Autodesk Inventor part; units mm, degrees
ref_plane "YZ Plane" through (0, 0, 0) normal (1, 0, 0) x (0, 1, 0)
ref_plane "XZ Plane" through (0, 0, 0) normal (0, 1, 0) x (-1, 0, 0)
ref_plane "XY Plane" through (0, 0, 0) normal (0, 0, 1) x (1, 0, 0)
sketch "Skizze1" plane through (0, 0, 0) normal (0, 0, 1) x (1, 0, 0)
  line L0 (0, 0) -> (14, 0)
  line L1 (14, 0) -> (14, 14)
  line L2 (14, 14) -> (0, 14)
  line L3 (0, 14) -> (0, 0)
  circle A0 centre (7, 7) radius 3.05
  dimension "d0" = 14
  dimension "d1" = 14
  dimension "d2" = 6.1
  dimension "d3" = 7
  dimension "d4" = 7
extrude "Extrusion1" add sketch "Skizze1" along normal blind 10
sketch "Skizze2" plane through (0, 14, 0) normal (0, 1, 0) x (1, 0, 0)
  line L0 (-6, 4) -> (20, 4)
  line L1 (20, 4) -> (20, -14)
  line L2 (20, -14) -> (-6, -14)
  line L3 (-6, -14) -> (-6, 4)
  line L4 (14, 0) -> (0, 0)
  line L5 (0, 0) -> (0, -10)
  line L6 (14, -10) -> (0, -10)
  line L7 (14, 0) -> (14, -10)
  arc A0 (-1.5, 1) -> (-4.5, 1) centre (-3, 1) ccw
  arc A1 (-4.5, -11) -> (-1.5, -11) centre (-3, -11) ccw
  arc A2 (18.5, 1) -> (15.5, 1) centre (17, 1) ccw
  arc A3 (15.5, -11) -> (18.5, -11) centre (17, -11) ccw
  line L8 (-4.5, 1) -> (-4.5, -11)
  line L9 (-1.5, -11) -> (-1.5, 1)
  line L10 (15.5, -11) -> (15.5, 1)
  line L11 (18.5, -11) -> (18.5, 1)
  point P0 (0, 0)
  dimension "d7" = 6
  dimension "d8" = 6
  dimension "d9" = 4
  dimension "d10" = 4
  dimension "d11" = 3
  dimension "d12" = 3
  dimension "d13" = 3
  dimension "d14" = 3
  dimension "d15" = 3
  dimension "d16" = 3
  dimension "d17" = 3
  dimension "d18" = 3
  dimension "d19" = 3
  dimension "d20" = 3
  dimension "d21" = 3
  dimension "d22" = 3
extrude "Extrusion2" add sketch "Skizze2" along normal blind 4 contours L0 L1 L2 L3 | L7 L6 L5 L4
properties part number "Stehlager 6mm"
Verification items for the finished model (mm, model axes). A direction names the side the tool comes from. Coordinates: 2 decimals unless noted, no trailing zeros. Write each loop counter-clockwise with the first axis right and the second up, starting at its lowest first coordinate (ties: lowest second). Pieces come first, ordered by that corner, then holes. Notation, with made-up numbers: (-2, -19) - (12, -19) arc R14 cw to (12, -3) - close; hole circle Ø3 at (-27.5, -5.75). An arc over 180 degrees is marked (long way). One line per question, with ' | ' between items. Start each with the question number.
1. Section check D-D (z = -1.5). Enter the section's corners in (x, y), plus the area to 3 significant figures.
2. Material ranges on line 1 along X through (y, z) = (16.25, 5.5); line 2 along Y through (x, z) = (7, 5.25); line 3 along X through (y, z) = (15.25, -2), recorded low to high.
3. Section check B-B (y = 7). Enter the section's corners in (x, z), plus the area to 3 significant figures.
4. Section check A-A (z = 3.75). Enter the section's corners in (x, y), plus the area to 3 significant figures.
5. Section check C-C (x = -3). Enter the section's corners in (y, z), plus the area to 3 significant figures.
6. Gauge pin test, flat ends, axial feed: P1, Ø8, axis at y = 8.5, z = 7, coming from the -X side; P2, Ø10, axis at x = 7, y = 7, coming from the -Z side; P3, Ø3, axis at y = 7, z = 2.5, coming from the +X side. Record the tip position at first contact, or that the pin passes through.
7. Access from +Z, -Z, +X, -X, +Y, -Y to the whole of each face (thin tool, end or side, straight path). Record for faces 1 (the flat face through (0, 7, 5)), 2 (the flat face through (3.8, 7.1, 0)), 3 (the flat face through (14, 7, 5)), 4 (the flat face through (18.5, 16, 5)).
8. Draft check along Z on faces 5 (the flat face through (7, 18, 5)), 6 (the flat face through (3.8, 7.1, 10)), 7 (the flat face through (15.5, 16, 5)). Enter one of: released by +Z, released by -Z, zero draft, split by the parting line, or undercut.
Computed values:
1) outline: (-6, 14) - (-4.41, 14) - (-4.41, 18) - (-6, 18) - close; (-1.59, 14) - (15.59, 14) - (15.59, 18) - (-1.59, 18) - close; (18.41, 14) - (20, 14) - (20, 18) - (18.41, 18) - close | area: 81.4 mm²
2) line 1: -6 to -4.5, -1.5 to 15.5, 18.5 to 20 | line 2: 0 to 3.95, 10.05 to 18 | line 3: -6 to -4.12, -1.88 to 15.88, 18.12 to 20
3) outline: (0, 0) - (3.95, 0) - (3.95, 10) - (0, 10) - close; (10.05, 0) - (14, 0) - (14, 10) - (10.05, 10) - close | area: 79.0 mm²
4) outline: (-6, 14) - (-4.5, 14) - (-4.5, 18) - (-6, 18) - close; (-1.5, 14) - (0, 14) - (0, 0) - (14, 0) - (14, 14) - (15.5, 14) - (15.5, 18) - (-1.5, 18) - close; (18.5, 14) - (20, 14) - (20, 18) - (18.5, 18) - close; hole circle Ø6.1 at (7, 7) | area: 247 mm²
5) outline: (14, -4) - (18, -4) - (18, -2.5) - (14, -2.5) - close; (14, 12.5) - (18, 12.5) - (18, 14) - (14, 14) - close | area: 12.0 mm²
6) P1: x = 0 | P2: z = 0 | P3: x = 14
7) face 1: +Z, -Z, -X, -Y | face 2: -Z, +X, -X, -Y | face 3: +Z, -Z, +X, -Y | face 4: +Y, -Y
8) face 5: zero draft | face 6: released by +Z | face 7: undercut
